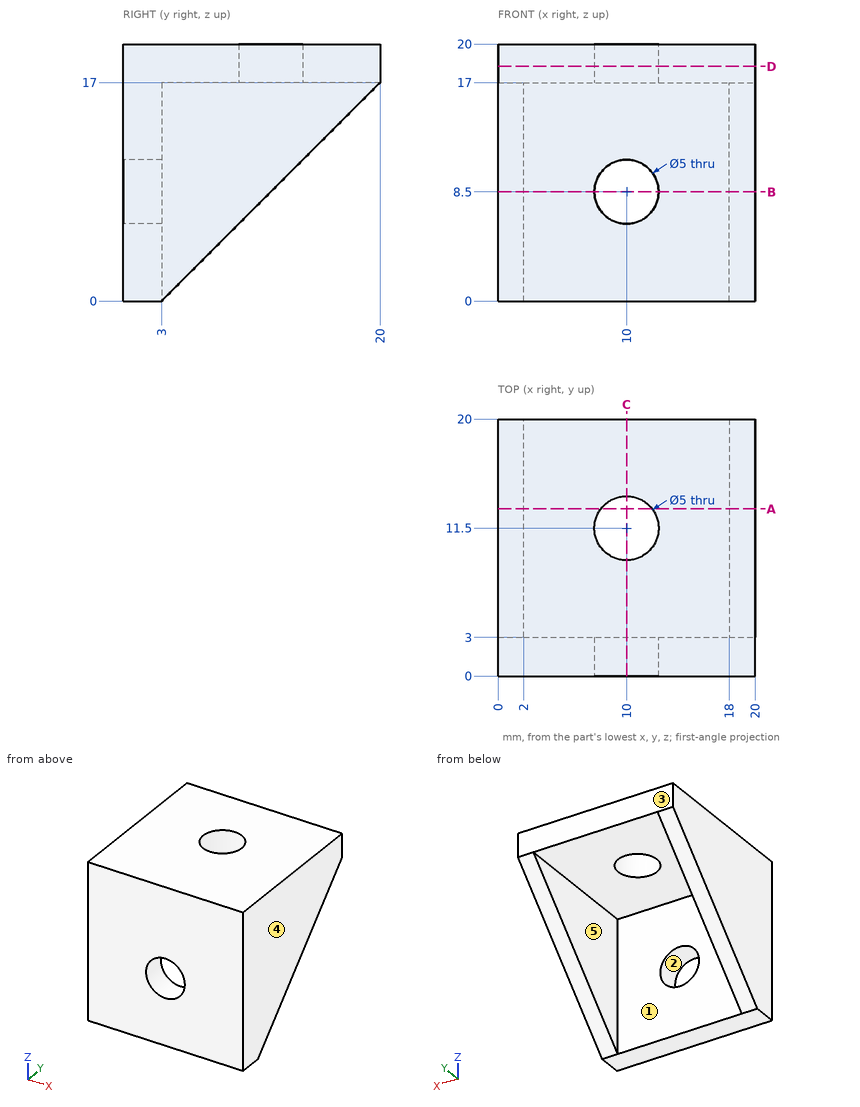
Answer from the drawing. Dimensions are ordinates in mm from the lowest x, y and z of the part. A direction names the side the tool comes from. Coordinates: 2 decimals unless noted, no trailing zeros. Write each loop counter-clockwise with the first axis right and the second up, starting at its lowest first coordinate (ties: lowest second). Pieces come first, ordered by that corner, then holes. Notation, with made-up numbers: M 39,85 L 71,85 A16 cw 71,111 Z; hole C 79,-22.5 d8. An arc over 180 degrees is marked long. Use one line per item in the form item = value. Start each with the question number.
1. A tool of negligible diameter and unlimited length cuts with its end or side. For the marked faces 1 and 2, from which of +Z, -Z, +X, -X, +Y, -Y can it reach the whole face along a straight path? Write none if from no direction.
2. Straight lines are drawn through the part: probe 1 along Y at (x, z) = (10, 19.4); probe 2 along X at (y, z) = (9.5, 11); probe 3 along X at (y, z) = (11.5, 19.05). For each, find the intervals that lie inside material, in ascending order. Write a range as from..to.
3. The part is cut by section D-D (z = 18.25). Give the vertices of the cut face in (x, y).
4. The part is cut by section A-A (y = 13). Give the vertices of the cut face in (x, z), plus the area to 3 significant figures.
5. Each of these flat-tipped pins is pushed along its axis until it touches: P1, Ø2, axis at x = 16.5, y = 5.5, coming from the -Z side; P2, Ø4, axis at x = 10, z = 8.5, coming from the +Y side; P3, Ø3, axis at x = 7.5, z = 10.5, coming from the +Y side; P4, Ø8, axis at x = 17, z = 2.5, coming from the +Y side. Where does it stop, or does it pass through?
6. The part is cut by section B-B (z = 8.5). Give the vertices of the cut face in (x, y), plus the area to 3 significant figures.
7. The part is cut by section C-C (x = 10). Give the vertices of the cut face in (y, z), plus the area to 3 significant figures.
8. The mould has two halves that part along X. Classify the marked faces 3, 4 and 5: released by +X, released by -X, zero draft, split by the parting line, or undercut.
Evaluation:
q1.face_1 = -Z, +Y
q1.face_2 = +Y, -Y
q2.probe_1 = 0..9, 14..20
q2.probe_2 = 0..2, 18..20
q2.probe_3 = 0..7.5, 12.5..20
q3.outline = M 0,0 L 20,0 L 20,20 L 0,20 Z; hole C 10,11.5 d5
q4.outline = M 0,10 L 2,10 L 2,17 L 8,17 L 8,20 L 0,20 Z; M 12,17 L 18,17 L 18,10 L 20,10 L 20,20 L 12,20 Z
q4.area = 76.0 mm^2
q5.P1 = 17
q5.P2 = through
q5.P3 = 3
q5.P4 = 9.37
q6.outline = M 0,0 L 7.5,0 L 7.5,3 L 2,3 L 2,11.5 L 0,11.5 Z; M 12.5,0 L 20,0 L 20,11.5 L 18,11.5 L 18,3 L 12.5,3 Z
q6.area = 79.0 mm^2
q7.outline = M 0,0 L 3,0 L 3,6 L 0,6 Z; M 0,11 L 3,11 L 3,17 L 9,17 L 9,20 L 0,20 Z; M 14,17 L 20,17 L 20,20 L 14,20 Z
q7.area = 81.0 mm^2
q8.face_3 = zero draft
q8.face_4 = released by +X
q8.face_5 = undercut
